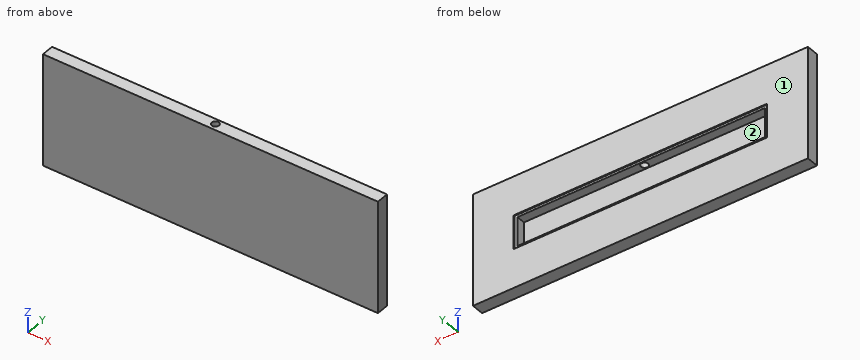
from build123d import *

# Parameters (mm, degrees)
SKETCH19_W               = 1135.16
SKETCH19_H               = 151.52
SKETCH19_W_2             = 1110
SKETCH19_H_2             = 130
BOSS_EXTRUDE2_DEPTH      = 40
SKETCH22_W               = 1135.16
SKETCH22_H               = 151.52
BOSS_EXTRUDE3_DEPTH      = 10
BOSS_EXTRUDE4_DEPTH      = 45
BOSS_EXTRUDE4_DEPTH_BACK = 10
SKETCH23_W               = 1500
SKETCH23_H               = 500
SKETCH23_W_2             = 1135.16
SKETCH23_H_2             = 151.52
SKETCH21_R               = 16
CUT_EXTRUDE5_DEPTH       = 792.849101786


with BuildPart() as part:
    # Sketch19 → Boss-Extrude2 (new body)
    with BuildSketch(Plane(origin=(0, 0, 0), x_dir=(1, 0, 0), z_dir=(0, 1, 0))):
        Rectangle(SKETCH19_W, SKETCH19_H)
        Rectangle(SKETCH19_W_2, SKETCH19_H_2, mode=Mode.SUBTRACT)
    extrude(amount=BOSS_EXTRUDE2_DEPTH)

    # Sketch22 → Boss-Extrude3 (add)
    with BuildSketch(Plane(origin=(0, 0, 0), x_dir=(1, 0, 0), z_dir=(0, 1, 0))):
        Rectangle(SKETCH22_W, SKETCH22_H)
    extrude(amount=-BOSS_EXTRUDE3_DEPTH)

    # Sketch23 → Boss-Extrude4 (add, two sides: drawn at the far end of the back side and taken through both)
    with BuildSketch(Plane(origin=(0, 0, 0), x_dir=(1, 0, 0), z_dir=(0, 1, 0)).offset(-BOSS_EXTRUDE4_DEPTH_BACK)):
        Rectangle(SKETCH23_W, SKETCH23_H)
        Rectangle(SKETCH23_W_2, SKETCH23_H_2, mode=Mode.SUBTRACT)
    extrude(amount=BOSS_EXTRUDE4_DEPTH + BOSS_EXTRUDE4_DEPTH_BACK)

    # Sketch21 → Cut-Extrude5 (cut, through all)
    with BuildSketch(Plane.XY):
        with Locations(Location((0, 20, 0), (0, 0, 180))):
            Circle(SKETCH21_R)
    extrude(amount=CUT_EXTRUDE5_DEPTH, mode=Mode.SUBTRACT)


solid = part.part
CAD build for the part. Positions are in the model's coordinates, mm. Face numbers are marked on the shaded views. Coordinates: 2 decimals unless noted, no trailing zeros. Order: outer loops, then holes, each group sorted by start corner. A loop starts at its lowest first (then second) coordinate and runs counter-clockwise, first axis right, second up. Notation, with made-up numbers: (-21.75, -13) -> (37.25, -13) arc R35 ccw to (37.25, 23) -> close; hole circle Ø4 at (89, 34.5). An arc over 180 degrees is marked (long way). Answer in a Markdown table with one row per item.
1) Band-saw the part on B-B (y = 20). List the corners of the cut face in (x, z).
Check values:
| item | result |
|---|---|
| outline | (-750, -250) -> (750, -250) -> (750, 250) -> (16, 250) -> (16, 65) -> (555, 65) -> (555, -65) -> (-555, -65) -> (-555, 65) -> (-16, 65) -> (-16, 250) -> (-750, 250) -> close |
2) Band-saw the part on C-C (z = 20.5). List the corners of the cut face in (x, y), and give its area (3 significant figures).
Check values:
| item | result |
|---|---|
| outline | (-750, -10) -> (750, -10) -> (750, 45) -> (567.58, 45) -> (567.58, 40) -> (555, 40) -> (555, 0) -> (-555, 0) -> (-555, 40) -> (-567.58, 40) -> (-567.58, 45) -> (-750, 45) -> close |
| area | 32,400 mm2 |
3) Mould opens along X. For the marked faces 1 and 2 say: pulls with the +X half, pulls with the -X half, needs draft (parallel to the pull), parting line crosses it, or undercut.
Check values:
| item | result |
|---|---|
| face 1 | needs draft |
| face 2 | undercut |
4) Band-saw the part on A-A (x = 0). List the corners of the cut face in (y, z).
Check values:
| item | result |
|---|---|
| outline | (-10, -250) -> (45, -250) -> (45, -75.76) -> (40, -75.76) -> (40, -65) -> (0, -65) -> (0, 65) -> (4, 65) -> (4, 250) -> (-10, 250) -> close; (36, 65) -> (40, 65) -> (40, 75.76) -> (45, 75.76) -> (45, 250) -> (36, 250) -> close |
5) Drill centre lines: line 1 (Z direction, x = -194.5, y = 39); line 2 (Z direction, x = -20.5, y = 42); line 3 (Y direction, x = 0, z = 190). Where is each one in solid material? Low to high.
Check values:
| item | result |
|---|---|
| line 1 | -250 to -65, 65 to 250 |
| line 2 | -250 to -75.76, 75.76 to 250 |
| line 3 | -10 to 4, 36 to 45 |
